The model under review builds one solid part; all positions refer to its coordinate system, in mm. A direction names the side the tool comes from. Coordinates: 2 decimals unless noted, no trailing zeros. Order: outer loops, then holes, each group sorted by start corner. A loop starts at its lowest first (then second) coordinate and runs counter-clockwise, first axis right, second up. Notation, with made-up numbers: M -28,14 L 30,14 A28 cw 30,34 Z; hole C -15.5,5.5 d10. An arc over 180 degrees is marked long. Answer as CSV lines item,"result". Start each with the question number.
Q1. For P1, Ø4.5, axis at x = -13.47, z = -13.47, coming from the +Y side; P2, Ø1, axis at y = 3.5, z = 2.5, coming from the +X side; P3, Ø3, axis at y = 2, z = 3, coming from the +X side; P4, Ø3, axis at x = -19.05, z = 0, coming from the +Y side, all flat-tipped, find the tip position at first contact; note any pin that passes through.
Q2. Machinability: for faces 5 (the face through (2, 6.762, 0)), 6 (the face through (1, 2, 0)), which of the approach directions +Z, -Z, +X, -X, +Y, -Y give a long, thin tool a straight path to every point of the face, cutting with its end or side? Answer none if there is none.
Q3. Consider section A-A on x = 0. Write out the cut boundary in (y, z) (1 decimal), and give its area (3 significant figures).
Q4. Consider section C-C on y = 5.25. Write out the cut boundary in (x, z) (1 decimal).
Q5. Wall thickness on L1, parallel to X at y = 1.4, z = 0 (3 decimals); L2, parallel to Y at x = 8.5, z = -8.5; L3, parallel to Z at x = 10, y = 0.5: over which ranges is each line inside the solid? List them lowest first. Write a range as [from, to].
Q6. Consider section B-B on z = 19.05. Write out the cut boundary in (x, y).
Q7. Consider section D-D on x = 19.05. Write out the cut boundary in (y, z).
Q8. The part is to be moulded in two halves that separate along X. For faces 1 (the face through (3.874, 5.153, 0.86)), 2 (the face through (0.534, 1.014, 20.746)), 3 (the face through (-1.08, 1.01, -20.46)), 4 (the face through (-5, 2, 5)), say which applies: +X half, -X half, draft (parallel to the pull), parting line (faces both ways), or undercut.
from build123d import *

# Parameters (mm, degrees)
SKETCH1_R           = 22.225
BOSS_EXTRUDE1_DEPTH = 2
SKETCH2_R           = 1.778
CUT_EXTRUDE1_DEPTH  = 32.494463799
SKETCH3_R           = 3.96875
BOSS_EXTRUDE2_DEPTH = 4.7625
SKETCH4_R           = 1.5875
CUT_EXTRUDE2_DEPTH  = 4.7625
FILLET1_R           = 1.5875
SKETCH5_R           = 0.79375
CUT_EXTRUDE6_DEPTH  = 2.54


with BuildPart() as part:
    # Sketch1 → Boss-Extrude1 (new body)
    with BuildSketch(Plane(origin=(0, 0, 0), x_dir=(1, 0, 0), z_dir=(0, 1, 0))):
        with Locations(Location((0, 0, 0), (0, 0, 270))):
            Circle(SKETCH1_R)
    extrude(amount=BOSS_EXTRUDE1_DEPTH)

    # Sketch2 → Cut-Extrude1 (cut, through all)
    with BuildSketch(Plane(origin=(0, 2, 0), x_dir=(1, 0, 0), z_dir=(0, 1, 0))):
        with Locations(Location((0, 19.05, 0), (0, 0, 270))):
            Circle(SKETCH2_R)
        with Locations(Location((13.470384182, 13.470384182, 0), (0, 0, 270))):
            Circle(SKETCH2_R)
        with Locations(Location((19.05, 0, 0), (0, 0, 270))):
            Circle(SKETCH2_R)
        with Locations(Location((13.470384182, -13.470384182, 0), (0, 0, 270))):
            Circle(SKETCH2_R)
        with Locations(Location((0, -19.05, 0), (0, 0, 270))):
            Circle(SKETCH2_R)
        with Locations(Location((-13.470384182, -13.470384182, 0), (0, 0, 270))):
            Circle(SKETCH2_R)
        with Locations(Location((-19.05, 0, 0), (0, 0, 270))):
            Circle(SKETCH2_R)
        with Locations(Location((-13.470384182, 13.470384182, 0), (0, 0, 270))):
            Circle(SKETCH2_R)
    extrude(amount=-CUT_EXTRUDE1_DEPTH, mode=Mode.SUBTRACT)

    # Sketch3 → Boss-Extrude2 (add)
    with BuildSketch(Plane(origin=(0, 2, 0), x_dir=(1, 0, 0), z_dir=(0, 1, 0))):
        with Locations(Location((0, 0, 0), (0, 0, 90))):
            Circle(SKETCH3_R)
    extrude(amount=BOSS_EXTRUDE2_DEPTH)

    # Sketch4 → Cut-Extrude2 (cut)
    with BuildSketch(Plane(origin=(0, 6.7625, 0), x_dir=(1, 0, 0), z_dir=(0, 1, 0))):
        with Locations(Location((0, 0, 0), (0, 0, 270))):
            Circle(SKETCH4_R)
    extrude(amount=-CUT_EXTRUDE2_DEPTH, mode=Mode.SUBTRACT)

    # Fillet1
    fillet1_edges = [part.edges().sort_by_distance(p)[0] for p in [
        (0, 2, 3.96875),
    ]]
    fillet(fillet1_edges, radius=FILLET1_R)

    # Sketch5 → Cut-Extrude6 (cut)
    with BuildSketch(Plane(origin=(0, 0, 0), x_dir=(-1, 0, 0), z_dir=(0, -1, 0))):
        with Locations(Location((0, 0, 0), (0, 0, 90))):
            Circle(SKETCH5_R)
    extrude(amount=-CUT_EXTRUDE6_DEPTH, mode=Mode.SUBTRACT)


solid = part.part
Evaluation:
1,P1,"stops at y = 2"
1,P2,"stops at x = 3.44"
1,P3,"stops at x = 22.17"
1,P4,"passes through"
2,face 5,"+Z, -Z, +X, -X, +Y"
2,face 6,"+Y"
3,outline,"M 0,-22.2 L 2,-22.2 L 2,-20.8 L 0,-20.8 Z; M 0,-17.3 L 2,-17.3 L 2,-5.6 A1.6 cw 3.6,-4 L 6.8,-4 L 6.8,-1.6 L 2,-1.6 L 2,-0.8 L 0,-0.8 Z; M 0,0.8 L 2,0.8 L 2,1.6 L 6.8,1.6 L 6.8,4 L 3.6,4 A1.6 cw 2,5.6 L 2,17.3 L 0,17.3 Z; M 0,20.8 L 2,20.8 L 2,22.2 L 0,22.2 Z"
3,area,"95.3 mm²"
4,outline,"C 0,0 d7.9; hole C 0,0 d3.2"
5,L1,"x = [-22.225, -20.828], [-17.272, -0.794], [0.794, 17.272], [20.828, 22.225]"
5,L2,"y = [0, 2]"
5,L3,"z = [-19.85, 19.85]"
6,outline,"M -11.45,0 L -1.78,0 L -1.78,2 L -11.45,2 Z; M 1.78,0 L 11.45,0 L 11.45,2 L 1.78,2 Z"
7,outline,"M 0,-11.45 L 2,-11.45 L 2,-1.78 L 0,-1.78 Z; M 0,1.78 L 2,1.78 L 2,11.45 L 0,11.45 Z"
8,face 1,"parting line"
8,face 2,"undercut"
8,face 3,"undercut"
8,face 4,"draft"
